Autodesk Inventor part; units mm, degrees
ref_plane "YZ Plane" through (0, 0, 0) normal (1, 0, 0) x (0, 1, 0)
ref_plane "XZ Plane" through (0, 0, 0) normal (0, 1, 0) x (-1, 0, 0)
ref_plane "XY Plane" through (0, 0, 0) normal (0, 0, 1) x (1, 0, 0)
sketch "Sketch1" plane through (0, 0, 0) normal (0, 0, 1) x (1, 0, 0)
  arc A0 (-4.5, -2.1795) -> (-4.5, 2.1795) centre (0, 0) ccw construction
  line L0 (-4.5, 2.1795) -> (-4.5, -2.1795) construction
  arc A1 (-4.5, 2.1795) -> (-4.5, -2.1795) centre (0, 0) ccw construction
  arc A2 (-4.6, -2.2023) -> (-4.6, 2.2023) centre (0, 0) ccw
  line L1 (-4.6, -2.2023) -> (-4.6, 2.2023)
  circle A3 centre (0, 0) radius 8
  dimension "d0" = 10
  dimension "d1" = 4.359
  dimension "d2" = 0.1
  dimension "d3" = 16
extrude "Extrusion1" add sketch "Sketch1" along normal blind 4
sketch "Sketch2" plane through (0, 0, 0) normal (0, 0, -1) x (-1, 0, 0)
  circle A0 centre (1, 0) radius 7.9
  arc A1 (4.6, 2.2023) -> (4.6, -2.2023) centre (0, 0) ccw
  line L0 (4.6, -2.2023) -> (4.6, 2.2023)
  dimension "d6" = 15.8
  dimension "d7" = 1
extrude "Extrusion2" add sketch "Sketch2" along normal blind 4
sketch "Sketch5" plane through (0, 0, 4) normal (0, 0, 1) x (1, 0, 0)
  circle A0 centre (0, 0) radius 8
extrude "Extrusion5" cut sketch "Sketch5" against normal up to surface (4 mm away)
sketch "Sketch6" plane through (-1, 0, -4) normal (0, 0, -1) x (-1, 0, 0)
  circle A0 centre (-1, 0) radius 9
  arc A1 (3.6, 2.2023) -> (3.6, -2.2023) centre (-1, 0) ccw
  line L0 (3.6, 2.2023) -> (3.6, -2.2023)
  dimension "d19" = 18
extrude "Extrusion6" add sketch "Sketch6" along normal blind 4.2
sketch "Sketch7" plane through (0, 0, -8.2) normal (0, 0, -1) x (-1, 0, 0)
  circle A0 centre (-1, 0) radius 7.9
  arc A1 (4.6, 2.2023) -> (4.6, -2.2023) centre (0, 0) ccw
  line L0 (4.6, 2.2023) -> (4.6, -2.2023)
  dimension "d22" = 15.8
  dimension "d23" = 1
extrude "Extrusion7" add sketch "Sketch7" along normal blind 4
properties part number "EccentricBearingShaft"
Geometry check sheet. Reference: the model listing, model coordinates, mm. A direction names the side the tool comes from. Round coordinates to 2 decimals unless told otherwise and drop trailing zeros. Order: outer loops, then holes, each group sorted by start corner. A loop starts at its lowest first (then second) coordinate and runs counter-clockwise, first axis right, second up. Notation, with made-up numbers: (-14, 73.25) -> (-1, 73.25) arc R23 cw to (-1, 98.25) -> close; hole circle Ø7 at (56, -2.75). An arc over 180 degrees is marked (long way). Use one line per item in the form item = value.
1. Cross-section at A-A, the plane y = 0. Enter the section's corners in (x, z).
Working result:
outline = (-9, -8.2) -> (-6.9, -8.2) -> (-6.9, -12.2) -> (-4.6, -12.2) -> (-4.6, 0) -> (-8.9, 0) -> (-8.9, -4) -> (-9, -4) -> close; (5.1, -12.2) -> (8.9, -12.2) -> (8.9, -8.2) -> (9, -8.2) -> (9, -4) -> (6.9, -4) -> (6.9, 0) -> (5.1, 0) -> close
2. Scan lines: line 1 along Y through (x, z) = (0, -6.5); line 2 along X through (y, z) = (0, -3.5); line 3 along Z through (x, y) = (-1.75, 8). Record each from-to range of solid material in increasing order. Write a range as from..to.
Working result:
line_1 = -9..-5.1, 5.1..9
line_2 = -8.9..-4.6, 5.1..6.9
line_3 = -8.2..-4
3. Set-up check for faces 1 (the face through (1.172, -8.923, -6.071)), 2 (the face through (-6.535, -2.373, -10.172)): record each of +Z, -Z, +X, -X, +Y, -Y from which the full face is reachable in a straight line by a thin tool's end or side.
Working result:
face_1 = +Z, -Z
face_2 = -Z
4. Cross-section at B-B, the plane x = -1. Enter the section's corners in (y, z), plus the area to 3 significant figures.
Working result:
outline = (-8.94, -8.2) -> (-7.64, -8.2) -> (-7.64, -12.2) -> (-5, -12.2) -> (-5, 0) -> (-7.9, 0) -> (-7.9, -4) -> (-8.94, -4) -> close; (5, -12.2) -> (7.64, -12.2) -> (7.64, -8.2) -> (8.94, -8.2) -> (8.94, -4) -> (7.9, -4) -> (7.9, 0) -> (5, 0) -> close
area = 77.4 mm^2
5. Cross-section at D-D, the plane y = 6.75. Enter the section's corners in (x, z), plus the area to 3 significant figures.
Working result:
outline = (-5.95, -8.2) -> (-3.1, -8.2) -> (-3.1, -12.2) -> (5.1, -12.2) -> (5.1, -8.2) -> (5.95, -8.2) -> (5.95, -4) -> (3.1, -4) -> (3.1, 0) -> (-5.1, 0) -> (-5.1, -4) -> (-5.95, -4) -> close
area = 116 mm^2
6. Cross-section at C-C, the plane z = -10. Enter the section's corners in (x, y), plus the area to 3 significant figures.
Working result:
outline = circle Ø15.8 at (1, 0); hole (-4.6, -2.2) arc R5.1 ccw (long way) to (-4.6, 2.2) -> close
area = 116 mm^2
7. Go/stop test with flat-tipped pins: pin 1 (9 mm diameter, centred on x = 0, y = 0, fed in from +Z); pin 2 (1 mm diameter, centred on y = -3, z = -6, fed in from +X); pin 3 (4 mm diameter, centred on y = 6.5, z = -3, fed in from -X); pin 4 (5 mm diameter, centred on x = -3.5, z = -7, fed in from +Y). Record where each tip stops, or that it passes through.
Working result:
pin_1 = through
pin_2 = 8.65
pin_3 = -7.63
pin_4 = 8.94
8. Mould release check, pull along X, two halves, no side actions. Record for faces 3 (the face through (7, -2, -4)), 4 (the face through (-5.25, -6.66, -1.97)), 5 (the face through (-4.6, 0, -6)): pulls with the +X half, pulls with the -X half, needs draft (parallel to the pull), parting line crosses it, or undercut.
Working result:
face_3 = needs draft
face_4 = parting line crosses it
face_5 = undercut
